Design review of the part built by this model. Coordinates are the model's own, in mm. A direction names the side the tool comes from. Coordinates: 2 decimals unless noted, no trailing zeros. Order: outer loops, then holes, each group sorted by start corner. A loop starts at its lowest first (then second) coordinate and runs counter-clockwise, first axis right, second up. Notation, with made-up numbers: M 79,-30.5 L 116,-30.5 A25 ccw 116,4.5 Z; hole C 77,-0.75 d1. An arc over 180 degrees is marked long. Answer in a Markdown table with one row per item.
from build123d import *

# Parameters (mm, degrees)
F0_W     = 546
F0_H     = 290
F1_DEPTH = 20
F2_W     = 521.951318
F2_H     = 262.995124
F3_DEPTH = 10
F4_R     = 7.5
F5_DEPTH = 30


with BuildPart() as f1:
    # F0 (on Front) → F1 (new body)
    with BuildSketch(Plane.XZ):
        Rectangle(F0_W, F0_H)
    extrude(amount=F1_DEPTH)

    # F2 (on face) → F3 (join)
    with BuildSketch(Plane.XZ.offset(20)):
        Rectangle(F2_W, F2_H)
    extrude(amount=F3_DEPTH)

    # F4 (on face) → F5 (join)
    with BuildSketch(Plane.XZ.offset(30)):
        with Locations((-74.205883, 0)):
            Circle(F4_R)
        with Locations((74.717641, 0)):
            Circle(F4_R)
    extrude(amount=F5_DEPTH)


solid = f1.part
(1) For line 1 along Y through (x, z) = (170.5, -99.5); line 2 along Z through (x, y) = (-208, -25); line 3 along X through (y, z) = (-26, -47), list the stretches that pass through material, from the lowest coordinate up. Write a range as from..to.
Return value:
| item | result |
|---|---|
| line 1 | y = -30..0 |
| line 2 | z = -131.5..131.5 |
| line 3 | x = -260.98..260.98 |
(2) Insertion check: pin 1 Ø8 at (x, y) = (-10.5, -24.5) entering from +Z; pin 2 Ø3 at (x, z) = (-184.5, -78.5) entering from +Y; pin 3 Ø4 at (x, z) = (-5, -44) entering from -Y; pin 4 Ø5 at (y, z) = (-23, 24) entering from -X. Each pin has a flat end and moves straight along its axis. Give the tip position at first contact, or say it passes through.
Return value:
| item | result |
|---|---|
| pin 1 | stops at z = 131.5 |
| pin 2 | stops at y = 0 |
| pin 3 | stops at y = -30 |
| pin 4 | stops at x = -260.98 |
(3) Add section A-A, the plane z = 0. Give the boundary of the cut face in (x, y), and give its area (3 significant figures).
Return value:
| item | result |
|---|---|
| outline | M -273,-20 L -260.98,-20 L -260.98,-30 L -81.71,-30 L -81.71,-60 L -66.71,-60 L -66.71,-30 L 67.22,-30 L 67.22,-60 L 82.22,-60 L 82.22,-30 L 260.98,-30 L 260.98,-20 L 273,-20 L 273,0 L -273,0 Z |
| area | 17,000 mm2 |
(4) For faces 4 (the flat face through (-260.976, -25, -2)), 5 (the flat face through (-4, -25, -131.498)), 6 (the flat face through (260.976, -25, -2)), 7 (the cylindrical face through (-67.05, -44.79, 2.25)), list the 3-axis set-ups (+Z, -Z, +X, -X, +Y, -Y) from which the entire face can be reached by the end or side of a thin tool; tool diameter is ignored.
Return value:
| item | result |
|---|---|
| face 4 | +Z, -Z, -X, -Y |
| face 5 | -Z, +X, -X, -Y |
| face 6 | +Z, -Z, +X, -Y |
| face 7 | -Y |
(5) Draft analysis for pull direction X (two halves, no side actions). For faces 1 (the cylindrical face through (81.871, -44.79, 2.253)), 2 (the flat face through (-273, -10, -2)), 3 (the flat face through (-4, -25, 131.498)), state which applies: pulls with the +X half, pulls with the -X half, needs draft (parallel to the pull), parting line crosses it, or undercut.
Return value:
| item | result |
|---|---|
| face 1 | undercut |
| face 2 | pulls with the -X half |
| face 3 | needs draft |
(6) Add section B-B, the plane y = -51. Give the boundary of the cut face in (x, z), and give its area (3 significant figures).
Return value:
| item | result |
|---|---|
| outline | C -74.21,0 d15; C 74.72,0 d15 |
| area | 353 mm2 |
(7) Add section C-C, the plane x = -40.5. Give the boundary of the cut face in (y, z).
Return value:
| item | result |
|---|---|
| outline | M -30,-131.5 L -20,-131.5 L -20,-145 L 0,-145 L 0,145 L -20,145 L -20,131.5 L -30,131.5 Z |
